from build123d import *

# Parameters (mm, degrees)
F2_DEPTH = 5.55625
F1_R     = 5.55625
F3_DEPTH = 28.575


with BuildPart() as f2:
    # F0 (on Top) → F2 (new body)
    with BuildSketch(Plane.XY):
        Polygon((4.582718, 7.9375), (-4.582718, 7.9375), (-9.165436, 0), (-4.582718, -7.9375), (4.582718, -7.9375), (9.165436, 0), align=None)
    extrude(amount=F2_DEPTH)

    # F1 (on Top) → F3 (join)
    with BuildSketch(Plane.XY):
        with Locations((0, 0.394696)):
            Circle(F1_R)
    extrude(amount=-F3_DEPTH)


solid = f2.part
Source: CAD feature listing. Evaluate the final solid. Frame: model axes, mm. A direction names the side the tool comes from. Give positions to 0.01 mm unless a question says otherwise; leave off trailing zeros. Write each loop counter-clockwise with the first axis right and the second up, starting at its lowest first coordinate (ties: lowest second). Pieces come first, ordered by that corner, then holes. Notation, with made-up numbers: M 58,35.5 L 81,35.5 A25 cw 81,63.5 Z; hole C -27,79.25 d7. An arc over 180 degrees is marked long. Return JSON: item names as keys, results as strings. Group by question number.
1) Cut plane C-C, the plane z = -6.5. Output: boundary loops of the cut face in (x, y).
2) Cut plane D-D, the plane x = 6.5. Output: boundary loops of the cut face in (y, z), then the cut area to 3 significant figures.
3) Cut plane A-A, the plane x = 0. Output: boundary loops of the cut face in (y, z) (1 decimal), then the cut area to 3 significant figures.
4) Cut plane B-B, the plane y = 2.75. Output: boundary loops of the cut face in (x, z) (3 decimals).
5) Set-up query: faces 1 (the face through (-6.842, 4.024, 2.739)), 2 (the face through (2, -5, 0)). Return all of +Z, -Z, +X, -X, +Y, -Y with unobstructed straight access to the full face (end or side cutting, diameter ignored); none if empty.
6) Ray query, L1, parallel to Z at x = 1, y = -7; L2, parallel to X at y = 0.5, z = -12.5; L3, parallel to X at y = -3.75, z = -25. Return the intervals inside material, ascending.
7) First-contact query: pin 1 Ø8 at (x, z) = (-2.5, -15.5) entering from +Y; pin 2 Ø4 at (y, z) = (-3.5, -22) entering from -X; pin 3 Ø8 at (x, z) = (2, -5.5) entering from -Y. Flat tips, straight axial feed; report the tip coordinate or a pass-through.
Data:
{
 "1": {"outline": "C 0,0.39 d11.11"},
 "2": {"outline": "M -4.62,0 L 4.62,0 L 4.62,5.56 L -4.62,5.56 Z", "area": "51.3 mm²"},
 "3": {"outline": "M -7.9,0 L -5.2,0 L -5.2,-28.6 L 6,-28.6 L 6,0 L 7.9,0 L 7.9,5.6 L -7.9,5.6 Z", "area": "406 mm²"},
 "4": {"outline": "M -7.578,0 L -5.032,0 L -5.032,-28.575 L 5.032,-28.575 L 5.032,0 L 7.578,0 L 7.578,5.556 L -7.578,5.556 Z"},
 "5": {"face 1": "+Z, -Z, -X, +Y", "face 2": "-Z"},
 "6": {"L1": "z = 0 to 5.56", "L2": "x = -5.56 to 5.56", "L3": "x = -3.7 to 3.7"},
 "7": {"pin 1": "stops at y = 5.95", "pin 2": "stops at x = -5.22", "pin 3": "stops at y = -5.16"}
}
